Autodesk Inventor part; units mm, degrees
ref_plane "YZ Plane" through (0, 0, 0) normal (1, 0, 0) x (0, 1, 0)
ref_plane "XZ Plane" through (0, 0, 0) normal (0, 1, 0) x (-1, 0, 0)
ref_plane "XY Plane" through (0, 0, 0) normal (0, 0, 1) x (1, 0, 0)
sketch "Sketch1" plane through (0, 0, 0) normal (0, 0, 1) x (1, 0, 0)
  circle A0 centre (0, 0) radius 25
  dimension "d0" = 50
extrude "Extrusion1" add sketch "Sketch1" along normal blind 70
hole "Hole1" at (0, 0, 70) direction (0, 0, -1) diameter 36 depth 60 tip angle 118 countersink diameter 40 countersink angle 70
fillet "Fillet1" radius 2 1 edges at (0, 20, 70)
sketch "Sketch2" plane through (0, 0, 70) normal (0, 0, 1) x (1, 0, 0)
  point P0 (0, 0)
fillet "Fillet2" radius 10 1 edges at (-25, 0, 0)
fillet "Fillet3" radius 10 1 edges at (-25, 0, 70)
sketch3d "3D Sketch2"
properties part number "solenoid_looking_pot"
Work out the finished part from the listing and answer in its coordinate system (mm). Coordinates: 2 decimals unless noted, no trailing zeros. Write each loop counter-clockwise with the first axis right and the second up, starting at its lowest first coordinate (ties: lowest second). Pieces come first, ordered by that corner, then holes.
Q1. Find the intervals of material crossed by line 1 (Y direction, x = 0, z = 48); line 2 (X direction, y = -9.5, z = 30); line 3 (X direction, y = -0.5, z = 59.5) (3 decimals), in increasing order.
Q2. Determine the mould class of faces 1 (the face through (23.846, -7.509, 35.651)), 2 (the face through (15.252, -9.724, 67.269)), 3 (the face through (0, -3, 0)) for opening direction Y: released by +Y, released by -Y, zero draft, split by the parting line, or undercut.
Q3. A cutting plane is placed at A-A, the plane y = 0. Give the vertices of the cut face in (x, z), then the cut area to 3 significant figures.
Q4. A cutting plane is placed at C-C, the plane z = 5.5. Give the vertices of the cut face in (x, y).
Q5. Each of these flat-tipped pins is pushed along its axis until it touches: pin 1 Ø10 at (x, z) = (-11.5, 46) entering from +Y; pin 2 Ø1.5 at (x, y) = (-4.5, -19) entering from -Z; pin 3 Ø12 at (x, z) = (8.5, 16) entering from +Y. Where does it stop, or does it pass through?
Findings below:
1. line 1: y = -25 to -18, 18 to 25
1. line 2: x = -23.12 to -15.29, 15.29 to 23.12
1. line 3: x = -24.995 to -17.993, 17.993 to 24.995
2. face 1: split by the parting line
2. face 2: undercut
2. face 3: zero draft
3. outline: (-25, 10) arc R10 ccw to (-15, 0) - (-1.36, 0) - (-18, 10) - (-18, 67.14) - (-19.4, 69.15) arc R2 ccw to (-21.04, 70) arc R10 ccw to (-25, 62.03) - close; (1.36, 0) - (15, 0) arc R10 ccw to (25, 10) - (25, 62.03) arc R10 ccw to (21.04, 70) arc R2 ccw to (19.4, 69.15) - (18, 67.14) - (18, 10) - close
3. area: 1,080 mm2
4. outline: circle Ø47.86 at (0, 0); hole circle Ø21.02 at (0, 0)
5. pin 1: stops at y = 24.14
5. pin 2: stops at z = 0.74
5. pin 3: stops at y = 24.87
